from build123d import *

# Parameters (mm, degrees)
SKETCH_W     = 114
SKETCH_H     = 35
SKETCH_W_2   = 13
SKETCH_H_2   = 23
PAD_DEPTH    = 4
SKETCH001_W  = 4
SKETCH001_H  = 6
POCKET_DEPTH = 5


with BuildPart() as part:
    # Sketch → Pad (new body)
    with BuildSketch(Plane.XY):
        Rectangle(SKETCH_W, SKETCH_H)
        Rectangle(SKETCH_W_2, SKETCH_H_2, mode=Mode.SUBTRACT)
        with BuildLine():
            ThreePointArc((-40.139128, 10.054315), (-50.193443, 0), (-40.139128, -10.054315))
            Line((-40.139128, -10.054315), (-20, -10.054315))
            ThreePointArc((-20, -10.054315), (-9.945685, 0), (-20, 10.054315))
            Line((-20, 10.054315), (-40.139128, 10.054315))
        make_face(mode=Mode.SUBTRACT)
        with BuildLine():
            ThreePointArc((20, 10.054315), (9.945685, 0), (20, -10.054315))
            Line((20, -10.054315), (40.139128, -10.054315))
            ThreePointArc((40.139128, -10.054315), (50.193443, 0), (40.139128, 10.054315))
            Line((40.139128, 10.054315), (20, 10.054315))
        make_face(mode=Mode.SUBTRACT)
    extrude(amount=PAD_DEPTH)

    # Sketch001 (on Face18 of Pad) → Pocket (cut)
    with BuildSketch(Plane.XY.offset(4)):
        with Locations((-55, 14.5)):
            Rectangle(SKETCH001_W, SKETCH001_H)
        with Locations((-55, -14.5)):
            Rectangle(SKETCH001_W, SKETCH001_H)
        with Locations((55, -14.5)):
            Rectangle(SKETCH001_W, SKETCH001_H)
        with Locations((55, 14.5)):
            Rectangle(SKETCH001_W, SKETCH001_H)
    extrude(amount=-POCKET_DEPTH, mode=Mode.SUBTRACT)


solid = part.part
Source: CAD feature listing. Evaluate the final solid. Frame: model axes, mm. A direction names the side the tool comes from. Give positions to 0.01 mm unless a question says otherwise; leave off trailing zeros. Write each loop counter-clockwise with the first axis right and the second up, starting at its lowest first coordinate (ties: lowest second). Pieces come first, ordered by that corner, then holes. Notation, with made-up numbers: M 88.5,-26 L 128.5,-26 A13 ccw 128.5,-20 Z; hole C -7.75,38.25 d1. An arc over 180 degrees is marked long. Answer as a JSON object with one key per item and string values.
Q1. Cut plane C-C, the plane x = 5. Return the cut outline in (y, z), then the cut area to 3 significant figures.
Geometry check:
{"outline": "M -17.5,0 L -11.5,0 L -11.5,4 L -17.5,4 Z; M 11.5,0 L 17.5,0 L 17.5,4 L 11.5,4 Z", "area": "48.0 mm^2"}
Q2. Cut plane B-B, the plane z = 2.95. Return the cut outline in (x, y).
Geometry check:
{"outline": "M -57,-11.5 L -53,-11.5 L -53,-17.5 L 53,-17.5 L 53,-11.5 L 57,-11.5 L 57,11.5 L 53,11.5 L 53,17.5 L -53,17.5 L -53,11.5 L -57,11.5 Z; hole M -40.14,-10.05 L -20,-10.05 A10.05 ccw -20,10.05 L -40.14,10.05 A10.05 ccw Z; hole M -6.5,-11.5 L 6.5,-11.5 L 6.5,11.5 L -6.5,11.5 Z; hole M 20,-10.05 L 40.14,-10.05 A10.05 ccw 40.14,10.05 L 20,10.05 A10.05 ccw Z"}
Q3. Access query for faces 1 (the face through (-6.5, 0, 2)), 2 (the face through (-53, 14, 2)), 3 (the face through (53, 14, 2)), 4 (the face through (55, -11.5, 2)), 5 (the face through (-55, -11.5, 2)). Directions: +Z, -Z, +X, -X, +Y, -Y. A direction counts if a zero-diameter tool reaches every point of the face in a straight line with its end or side. Return the directions, or none.
Geometry check:
{"face 1": "+Z, -Z", "face 2": "+Z, -Z, -X, +Y", "face 3": "+Z, -Z, +X, +Y", "face 4": "+Z, -Z, +X, -Y", "face 5": "+Z, -Z, -X, -Y"}
Q4. Cut plane A-A, the plane y = 0. Return the cut outline in (x, z).
Geometry check:
{"outline": "M -57,0 L -50.19,0 L -50.19,4 L -57,4 Z; M -9.95,0 L -6.5,0 L -6.5,4 L -9.95,4 Z; M 6.5,0 L 9.95,0 L 9.95,4 L 6.5,4 Z; M 50.19,0 L 57,0 L 57,4 L 50.19,4 Z"}
Q5. Cut plane D-D, the plane y = 7.5. Return the cut outline in (x, z).
Geometry check:
{"outline": "M -57,0 L -46.84,0 L -46.84,4 L -57,4 Z; M -13.3,0 L -6.5,0 L -6.5,4 L -13.3,4 Z; M 6.5,0 L 13.3,0 L 13.3,4 L 6.5,4 Z; M 46.84,0 L 57,0 L 57,4 L 46.84,4 Z"}
Q6. Contact query for flat-ended pins moving along their axis: P1, Ø1.2, axis at x = 54, z = 1.5, coming from the +Y side; P2, Ø2, axis at x = -56, z = 1.5, coming from the -Y side; P3, Ø1.2, axis at y = -15, z = 1.5, coming from the +X side. Output: stop coordinate, or through.
Geometry check:
{"P1": "stops at y = 11.5", "P2": "stops at y = -11.5", "P3": "stops at x = 53"}
Q7. Ray query, line 1 along X through (y, z) = (0.5, 1.6); line 2 along Y through (x, z) = (-34.5, 1.7); line 3 along Y through (x, z) = (-4.5, 1). Return the intervals inside material, ascending.
Geometry check:
{"line 1": "x = -57 to -50.18, -9.96 to -6.5, 6.5 to 9.96, 50.18 to 57", "line 2": "y = -17.5 to -10.05, 10.05 to 17.5", "line 3": "y = -17.5 to -11.5, 11.5 to 17.5"}
Q8. Mould query, pull axis X, two halves, no side actions, for faces 6 (the face through (-1, 12, 4)), 7 (the face through (-57, 0, 2)), 8 (the face through (30, -10.054, 2)). Classes: +X half, -X half, draft (parallel to the pull), parting line (faces both ways), or undercut.
Geometry check:
{"face 6": "draft", "face 7": "-X half", "face 8": "undercut"}
